Source: CAD feature listing. Evaluate the final solid. Frame: model axes, mm. A direction names the side the tool comes from. Round coordinates to 2 decimals unless told otherwise and drop trailing zeros. Loops run counter-clockwise (first coordinate to the right, second up) from the corner with the lowest first, then second, coordinate; pieces in that order, holes last. Notation, with made-up numbers: (10, -14) - (26, -14) arc R32 cw to (26, 25) - close; hole circle Ø8 at (9, 61). An arc over 180 degrees is marked (long way). One line per question, with ' | ' between items.
from build123d import *

# Parameters (mm, degrees)
SKETCH1_W                 = 37
SKETCH1_H                 = 22.5
BOSS_EXTRUDE1_DEPTH       = 19
SKETCH2_W                 = 3.1
SKETCH2_H                 = 5.3
BOSS_EXTRUDE2_DEPTH       = 5.2
SKETCH3_R                 = 1.35
CUT_EXTRUDE1_DEPTH        = 46.050027747
FILLET1_R                 = 3.5
SKETCH4_R                 = 3.6
BOSS_EXTRUDE3_DEPTH       = 0.1
BOSS_EXTRUDE4_START       = 0.1
SKETCH5_R                 = 3.6
BOSS_EXTRUDE4_DEPTH       = 0.1
SKETCH6_R                 = 2.7
BOSS_EXTRUDE5_DEPTH       = 8.9
BOSS_EXTRUDE6_START       = 8.9
SKETCH7_R                 = 2.7
BOSS_EXTRUDE6_DEPTH       = 8.9
FILLET2_R                 = 0.5
CUT_EXTRUDE2_START        = -8.2
CUT_EXTRUDE2_DEPTH        = 8.2
CUT_EXTRUDE3_DEPTH        = 8.2
M2X0_4_TAPPED_HOLE1_D     = 1.6
M2X0_4_TAPPED_HOLE1_DEPTH = 5.2
M2X0_4_TAPPED_HOLE1_TIP   = 0.480688495
M2X0_4_TAPPED_HOLE2_D     = 1.6
M2X0_4_TAPPED_HOLE2_DEPTH = 5.2
M2X0_4_TAPPED_HOLE2_TIP   = 0.480688495
SKETCH16_R                = 1.95
BOSS_EXTRUDE7_DEPTH       = 2
BOSS_EXTRUDE8_DEPTH       = 11.5
SKETCH18_W                = 3.5
SKETCH18_H                = 5.2
BOSS_EXTRUDE9_DEPTH       = 2.5
SKETCH19_W                = 3.5
SKETCH19_H                = 5.2
BOSS_EXTRUDE10_DEPTH      = 2.5
BOSS_EXTRUDE11_DEPTH      = 13.5
FILLET3_R                 = 1.7
BOSS_EXTRUDE12_DEPTH      = 2
SKETCH23_W                = 3.2
SKETCH23_H                = 6.5
SKETCH23_H_2              = 8.5
CUT_EXTRUDE4_DEPTH        = 6
SKETCH25_R                = 1.45
CUT_EXTRUDE5_DEPTH        = 52.878728782
FILLET4_R                 = 0.5
SKETCH26_R                = 1
BOSS_EXTRUDE13_DEPTH      = 10


with BuildPart() as part:
    # Sketch1 → Boss-Extrude1 (new body)
    with BuildSketch(Plane(origin=(0, 0, 0), x_dir=(0, 0, -1), z_dir=(1, 0, 0))):
        with Locations((-18.5, 0)):
            Rectangle(SKETCH1_W, SKETCH1_H)
    extrude(amount=BOSS_EXTRUDE1_DEPTH)

    # Sketch2 → Boss-Extrude2 (add)
    with BuildSketch(Plane.XY.offset(37)):
        with Locations((9.5, 0)):
            Rectangle(SKETCH2_W, SKETCH2_H)
    extrude(amount=BOSS_EXTRUDE2_DEPTH)

    # Sketch3 → Cut-Extrude1 (cut, through all)
    with BuildSketch(Plane(origin=(11.05, 0, 0), x_dir=(0, 0, -1), z_dir=(1, 0, 0))):
        with Locations((-39.6, 0)):
            Circle(SKETCH3_R)
    extrude(amount=-CUT_EXTRUDE1_DEPTH, mode=Mode.SUBTRACT)

    # Fillet1
    fillet1_edges = [part.edges().sort_by_distance(p)[0] for p in [
        (9.5, -11.25, 37),
        (9.5, 11.25, 37),
    ]]
    fillet(fillet1_edges, radius=FILLET1_R)

    # Sketch4 → Boss-Extrude3 (add)
    with BuildSketch(Plane(origin=(19, 0, 0), x_dir=(0, 0, -1), z_dir=(1, 0, 0))):
        with Locations(Location((-25, 0, 0), (0, 0, 180))):
            Circle(SKETCH4_R)
    extrude(amount=BOSS_EXTRUDE3_DEPTH)

    # Sketch5 → Boss-Extrude4 (add)
    with BuildSketch(Plane.ZY.offset(BOSS_EXTRUDE4_START)):
        with Locations((25, 0)):
            Circle(SKETCH5_R)
    extrude(amount=-BOSS_EXTRUDE4_DEPTH)

    # Sketch6 → Boss-Extrude5 (add)
    with BuildSketch(Plane(origin=(19.1, 0, 0), x_dir=(0, 0, -1), z_dir=(1, 0, 0))):
        with Locations((-25, 0)):
            Circle(SKETCH6_R)
    extrude(amount=BOSS_EXTRUDE5_DEPTH)

    # Sketch7 → Boss-Extrude6 (add)
    with BuildSketch(Plane.ZY.offset(0.1).offset(BOSS_EXTRUDE6_START)):
        with Locations(Location((25, 0, 0), (0, 0, 180))):
            Circle(SKETCH7_R)
    extrude(amount=-BOSS_EXTRUDE6_DEPTH)

    # Fillet2
    fillet2_edges = [part.edges().sort_by_distance(p)[0] for p in [
        (9.5, 2.65, 37),
        (9.5, -2.65, 37),
    ]]
    fillet(fillet2_edges, radius=FILLET2_R)

    # Sketch8 → Cut-Extrude2 (cut)
    with BuildSketch(Plane(origin=(28, 0, 0), x_dir=(0, 0, -1), z_dir=(1, 0, 0)).offset(CUT_EXTRUDE2_START)):
        with BuildLine():
            Line((-26.8, -2.01246118), (-26.8, 2.01246118))
            ThreePointArc((-26.8, 2.01246118), (-27.7, 0), (-26.8, -2.01246118))
        make_face()
        with BuildLine():
            ThreePointArc((-22.3, 0), (-22.535248491, 1.102270384), (-23.2, 2.01246118))
            Line((-23.2, 2.01246118), (-23.2, -2.01246118))
            ThreePointArc((-23.2, -2.01246118), (-22.535248491, -1.102270384), (-22.3, 0))
        make_face()
    extrude(amount=CUT_EXTRUDE2_DEPTH, mode=Mode.SUBTRACT)

    # Sketch9 → Cut-Extrude3 (cut)
    with BuildSketch(Plane.ZY.offset(9)):
        with BuildLine():
            Line((23.2, -2.01246118), (23.2, 2.01246118))
            ThreePointArc((23.2, 2.01246118), (22.3, 0), (23.2, -2.01246118))
        make_face()
        with BuildLine():
            ThreePointArc((27.7, 0), (27.464751509, 1.102270384), (26.8, 2.01246118))
            Line((26.8, 2.01246118), (26.8, -2.01246118))
            ThreePointArc((26.8, -2.01246118), (27.464751509, -1.102270384), (27.7, 0))
        make_face()
    extrude(amount=-CUT_EXTRUDE3_DEPTH, mode=Mode.SUBTRACT)

    # M2x0.4 Tapped Hole1
    with Locations(Plane(origin=(28, 0, 0), x_dir=(0, 0, -1), z_dir=(1, 0, 0))):
        with Locations((-25, 0)):
            Hole(M2X0_4_TAPPED_HOLE1_D / 2, depth=M2X0_4_TAPPED_HOLE1_DEPTH)
            with Locations((0, 0, -(M2X0_4_TAPPED_HOLE1_DEPTH + M2X0_4_TAPPED_HOLE1_TIP / 2))):  # 118° drill point
                Cone(0, M2X0_4_TAPPED_HOLE1_D / 2, M2X0_4_TAPPED_HOLE1_TIP, mode=Mode.SUBTRACT)

    # M2x0.4 Tapped Hole2
    with Locations(Plane.ZY.offset(9)):
        with Locations((25, 0)):
            Hole(M2X0_4_TAPPED_HOLE2_D / 2, depth=M2X0_4_TAPPED_HOLE2_DEPTH)
            with Locations((0, 0, -(M2X0_4_TAPPED_HOLE2_DEPTH + M2X0_4_TAPPED_HOLE2_TIP / 2))):  # 118° drill point
                Cone(0, M2X0_4_TAPPED_HOLE2_D / 2, M2X0_4_TAPPED_HOLE2_TIP, mode=Mode.SUBTRACT)

    # Sketch16 → Boss-Extrude7 (add)
    with BuildSketch(Plane.ZY):
        with Locations((13.75, 0)):
            Circle(SKETCH16_R)
    extrude(amount=BOSS_EXTRUDE7_DEPTH)

    # Sketch17 → Boss-Extrude8 (add)
    with BuildSketch(Plane(origin=(0, 0, 0), x_dir=(-1, 0, 0), z_dir=(0, 0, -1))):
        with BuildLine():
            Line((-19, 6.025985397), (-19, -6.025985397))
            ThreePointArc((-19, -6.025985397), (-10.560588754, -11.199895156), (-1.3, -7.7021101))
            Line((-1.3, -7.7021101), (-1.3, 7.7021101))
            ThreePointArc((-1.3, 7.7021101), (-10.560588754, 11.199895156), (-19, 6.025985397))
        make_face()
    extrude(amount=BOSS_EXTRUDE8_DEPTH)

    # Sketch18 → Boss-Extrude9 (add)
    with BuildSketch(Plane(origin=(19, 0, 0), x_dir=(0, 0, -1), z_dir=(1, 0, 0))):
        with Locations((5.75, 0)):
            Rectangle(SKETCH18_W, SKETCH18_H)
    extrude(amount=BOSS_EXTRUDE9_DEPTH)

    # Sketch19 → Boss-Extrude10 (add)
    with BuildSketch(Plane.ZY.offset(-1.3)):
        with Locations((-5.75, 0)):
            Rectangle(SKETCH19_W, SKETCH19_H)
    extrude(amount=BOSS_EXTRUDE10_DEPTH)

    # Sketch20 → Boss-Extrude11 (add)
    with BuildSketch(Plane(origin=(0, 0, -11.5), x_dir=(-1, 0, 0), z_dir=(0, 0, -1))):
        with BuildLine():
            Line((-18, 5.728219619), (-18, -5.728219619))
            ThreePointArc((-18, -5.728219619), (-10.518083587, -10.199313987), (-2.3, -7.295375247))
            Line((-2.3, -7.295375247), (-2.3, 7.295375247))
            ThreePointArc((-2.3, 7.295375247), (-10.518083587, 10.199313987), (-18, 5.728219619))
        make_face()
    extrude(amount=BOSS_EXTRUDE11_DEPTH)

    # Fillet3
    fillet3_edges = [part.edges().sort_by_distance(p)[0] for p in [
        (10.518083587, 10.199313987, -25),
        (10.518083587, -10.199313987, -25),
    ]]
    fillet(fillet3_edges, radius=FILLET3_R)

    # Sketch21 → Boss-Extrude12 (add)
    with BuildSketch(Plane(origin=(0, 0, -25), x_dir=(-1, 0, 0), z_dir=(0, 0, -1))):
        with BuildLine():
            Line((-5.5, -3), (-5.5, 3))
            ThreePointArc((-5.5, 3), (-14.5, 0), (-5.5, -3))
        make_face()
    extrude(amount=BOSS_EXTRUDE12_DEPTH)

    # Sketch23 → Cut-Extrude4 (cut)
    with BuildSketch(Plane(origin=(0, 0, -25), x_dir=(-1, 0, 0), z_dir=(0, 0, -1))):
        with Locations((-9.5, 10.25)):
            Rectangle(SKETCH23_W, SKETCH23_H)
        with Locations((-9.5, -11.25)):
            Rectangle(SKETCH23_W, SKETCH23_H_2)
    extrude(amount=-CUT_EXTRUDE4_DEPTH, mode=Mode.SUBTRACT)

    # Sketch25 → Cut-Extrude5 (cut, through all)
    with BuildSketch(Plane(origin=(19, 0, 0), x_dir=(0, 0, -1), z_dir=(1, 0, 0))):
        with Locations((-4.95, 8.8)):
            Circle(SKETCH25_R)
        with Locations((-4.95, -8.8)):
            Circle(SKETCH25_R)
    extrude(amount=-CUT_EXTRUDE5_DEPTH, mode=Mode.SUBTRACT)

    # Fillet4
    fillet4_edges = [part.edges().sort_by_distance(p)[0] for p in [
        (0, -11.25, 16.75),
        (0, -10.224873734, 35.974873734),
        (0, 0, 37),
        (0, 10.224873734, 35.974873734),
        (19, -11.25, 16.75),
        (19, -10.224873734, 35.974873734),
        (19, 0, 37),
        (19, 10.224873734, 35.974873734),
        (0, 11.25, 16.75),
        (19, 11.25, 16.75),
    ]]
    fillet(fillet4_edges, radius=FILLET4_R)

    # Sketch26 → Boss-Extrude13 (add)
    with BuildSketch(Plane(origin=(0, 0, -27), x_dir=(-1, 0, 0), z_dir=(0, 0, -1))):
        with Locations((-9.5, 0)):
            Circle(SKETCH26_R)
    extrude(amount=BOSS_EXTRUDE13_DEPTH)


solid = part.part
1. Section query A-A, the plane z = 39.6. Return loops of the section in (x, y), plus the area to 3 significant figures.
Worked out:
outline: (7.95, -2.65) - (11.05, -2.65) - (11.05, -1.35) - (7.95, -1.35) - close; (7.95, 1.35) - (11.05, 1.35) - (11.05, 2.65) - (7.95, 2.65) - close | area: 8.06 mm2
2. Access query for faces 4 (the flat face through (7.9, -9, -22)), 5 (the flat face through (24, 0, 26.8)), 6 (the cylindrical face through (25.364, 0.24, 25.763)), 7 (the flat face through (0, 2.6, -6)), 8 (the flat face through (11.1, 9, -22)). Directions: +Z, -Z, +X, -X, +Y, -Y. A direction counts if a zero-diameter tool reaches every point of the face in a straight line with its end or side. Return the directions, or none.
Worked out:
face 4: -Z, -Y | face 5: +Z, +X, +Y, -Y | face 6: +X | face 7: -Z, -X, +Y | face 8: -Z, +Y
3. Section query D-D, the plane z = -1.5. Return loops of the section in (x, y).
Worked out:
outline: (1.3, -7.7) arc R11.25 ccw to (19, -6.03) - (19, 6.03) arc R11.25 ccw to (1.3, 7.7) - close
4. Material intervals for probe 1 along Z at (x, y) = (-7.4, 0); probe 2 along X at (y, z) = (-6, 30); probe 3 along Y at (x, z) = (-6.2, 25), sorted ascending.
Worked out:
probe 1: z = 23.2 to 24.2, 25.8 to 26.8 | probe 2: x = 0 to 19 | probe 3: y = -2.7 to -0.8, 0.8 to 2.7
5. Section query C-C, the plane x = 12.5. Give the number of separate pieces and of enclosed holes in the cut face, plus the area to 3 significant figures.
Worked out:
separate pieces: 1 | enclosed holes: 2 | area: 1,340 mm2
6. Section query B-B, the plane z = 29.5. Return loops of the section in (x, y), plus the area to 3 significant figures.
Worked out:
outline: (0, -10.75) arc R0.5 ccw to (0.5, -11.25) - (18.5, -11.25) arc R0.5 ccw to (19, -10.75) - (19, 10.75) arc R0.5 ccw to (18.5, 11.25) - (0.5, 11.25) arc R0.5 ccw to (0, 10.75) - close | area: 427 mm2
7. Mould query, pull axis X, two halves, no side actions, for faces 1 (the flat face through (10.1, -1, -27)), 2 (the flat face through (10, 9, -19)), 3 (the flat face through (19.1, -3, 26)). Classes: released by +X, released by -X, zero draft, split by the parting line, or undercut.
Worked out:
face 1: zero draft | face 2: undercut | face 3: released by +X
8. Contact query for flat-ended pins moving along their axis: P1, Ø10, axis at y = -2.5, z = -3, coming from the +X side; P2, Ø1.2, axis at x = 24, y = -0.5, coming from the -Z side; P3, Ø3, axis at y = -0.5, z = -5.5, coming from the -X side. Output: stop coordinate, or through.
Worked out:
P1: stops at x = 21.5 | P2: stops at z = 23.2 | P3: stops at x = -1.2
